Source: CAD feature listing. Evaluate the final solid. Frame: model axes, mm. Face numbers are marked on the shaded views. A direction names the side the tool comes from. Round coordinates to 2 decimals unless told otherwise and drop trailing zeros. Loops run counter-clockwise (first coordinate to the right, second up) from the corner with the lowest first, then second, coordinate; pieces in that order, holes last. Notation, with made-up numbers: M 51.25,75 L 99.25,75 A17 cw 99.25,105 Z; hole C 18.5,-18.5 d1. An arc over 180 degrees is marked long. Answer as a JSON object with one key per item and string values.
from build123d import *

# Parameters (mm, degrees)
SKETCH1_R           = 7
SKETCH1_R_2         = 5.2
BOSS_EXTRUDE1_DEPTH = 15.66
BOSS_EXTRUDE2_START = -2
SKETCH2_W           = 6
SKETCH2_H           = 4
BOSS_EXTRUDE2_DEPTH = 2
SKETCH4_R           = 1.5
CUT_EXTRUDE1_DEPTH  = 10
FILLET1_R           = 3
BOSS_EXTRUDE3_START = -1
SKETCH5_R           = 5.2
BOSS_EXTRUDE3_DEPTH = 1


with BuildPart() as part:
    # Sketch1 → Boss-Extrude1 (new body)
    with BuildSketch(Plane(origin=(0, 0, 0), x_dir=(1, 0, 0), z_dir=(0, 1, 0))):
        with Locations(Location((0, 0, 0), (0, 0, 270))):
            Circle(SKETCH1_R)
        with Locations(Location((0, 0, 0), (0, 0, 270))):
            Circle(SKETCH1_R_2, mode=Mode.SUBTRACT)
    extrude(amount=BOSS_EXTRUDE1_DEPTH)

    # Sketch2 → Boss-Extrude2 (add)
    with BuildSketch(Plane(origin=(0, 15.66, 0), x_dir=(1, 0, 0), z_dir=(0, 1, 0)).offset(BOSS_EXTRUDE2_START)):
        with Locations((-10.67, -9)):
            Rectangle(SKETCH2_W, SKETCH2_H)
        with BuildLine():
            ThreePointArc((0, -7), (-7, 0), (0, 7))
            Line((0, 7), (-7.67, 7))
            Line((-7.67, 7), (-13.67, 7))
            Line((-13.67, 7), (-13.67, -7))
            Line((-13.67, -7), (-7.67, -7))
            Line((-7.67, -7), (0, -7))
        make_face()
        with Locations((-10.67, 9)):
            Rectangle(SKETCH2_W, SKETCH2_H)
    extrude(amount=BOSS_EXTRUDE2_DEPTH)

    # Sketch4 → Cut-Extrude1 (cut)
    with BuildSketch(Plane.XZ.offset(-13.66)):
        with Locations(Location((-10.68, -8, 0), (0, 0, 270))):
            Circle(SKETCH4_R)
        with Locations(Location((-10.68, 8, 0), (0, 0, 270))):
            Circle(SKETCH4_R)
    extrude(amount=-CUT_EXTRUDE1_DEPTH, mode=Mode.SUBTRACT)

    # Fillet1
    fillet1_edges = [part.edges().sort_by_distance(p)[0] for p in [
        (-7.67, 14.66, 7),
        (-7.67, 14.66, -7),
    ]]
    fillet(fillet1_edges, radius=FILLET1_R)

    # Sketch5 → Boss-Extrude3 (add)
    with BuildSketch(Plane(origin=(0, 15.66, 0), x_dir=(1, 0, 0), z_dir=(0, 1, 0)).offset(BOSS_EXTRUDE3_START)):
        with Locations(Location((0, 0, 0), (0, 0, 270))):
            Circle(SKETCH5_R)
    extrude(amount=BOSS_EXTRUDE3_DEPTH)


solid = part.part
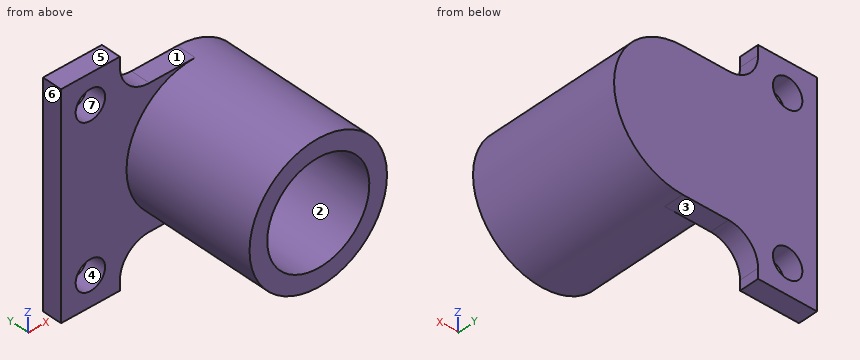
Item 1: Access query for the marked faces 1, 2 and 3. Directions: +Z, -Z, +X, -X, +Y, -Y. A direction counts if a zero-diameter tool reaches every point of the face in a straight line with its end or side. Return the directions, or none.
Answer sheet:
{"face 1": "+Z, +X, +Y, -Y", "face 2": "-Y", "face 3": "-Z, +X, +Y, -Y"}
Item 2: Contact query for flat-ended pins moving along their axis: pin 1 Ø4 at (x, z) = (-10.68, 8) entering from -Y; pin 2 Ø11 at (x, z) = (-8.5, -1) entering from -Y; pin 3 Ø0.8 at (y, z) = (14.5, 10.5) entering from +X; pin 4 Ø1 at (x, y) = (-2, 10.5) entering from +Z. Output: stop coordinate, or through.
Answer sheet:
{"pin 1": "stops at y = 13.66", "pin 2": "stops at y = 0", "pin 3": "stops at x = -7.67", "pin 4": "stops at z = 6.84"}
Item 3: Section B-B on z = 8. Return the cut outline in (x, y).
Answer sheet:
{"outline": "M -13.67,13.66 L -12.18,13.66 L -12.18,15.66 L -13.67,15.66 Z; M -9.18,13.66 L -6.91,13.66 L -6.91,15.66 L -9.18,15.66 Z"}
Item 4: Section C-C on y = 11.75. Return the cut outline in (x, z), then the cut area to 3 significant figures.
Answer sheet:
{"outline": "C 0,0 d14; hole C 0,0 d10.4", "area": "69.0 mm²"}
Item 5: Section D-D on z = 0. Return the cut outline in (x, y).
Answer sheet:
{"outline": "M -13.67,13.66 L -7,13.66 L -7,0 L -5.2,0 L -5.2,14.66 L 5.2,14.66 L 5.2,0 L 7,0 L 7,15.66 L -13.67,15.66 Z"}
Item 6: Section A-A on x = -10.68. Return the cut outline in (y, z), then the cut area to 3 significant figures.
Answer sheet:
{"outline": "M 13.66,-11 L 15.66,-11 L 15.66,-9.5 L 13.66,-9.5 Z; M 13.66,-6.5 L 15.66,-6.5 L 15.66,6.5 L 13.66,6.5 Z; M 13.66,9.5 L 15.66,9.5 L 15.66,11 L 13.66,11 Z", "area": "32.0 mm²"}
Item 7: Line query: probe 1 along Y at (x, z) = (-3.25, -3.75); probe 2 along Y at (x, z) = (-7, -3.25); probe 3 along Z at (x, y) = (-4, 11.25). Output: solid intervals per line, ascending. Write a range as from..to.
Answer sheet:
{"probe 1": "y = 14.66..15.66", "probe 2": "y = 13.66..15.66", "probe 3": "z = -5.74..-3.32, 3.32..5.74"}
Item 8: Pull-direction query (X, two-part tool) for the marked faces 4, 5, 6 and 7; classes: pulls with the +X half, pulls with the -X half, needs draft (parallel to the pull), parting line crosses it, or undercut.
Answer sheet:
{"face 4": "undercut", "face 5": "needs draft", "face 6": "pulls with the -X half", "face 7": "undercut"}
